Build history of the part. All positions in model axes, mm. A direction names the side the tool comes from. Round coordinates to 2 decimals unless told otherwise and drop trailing zeros. Write each loop counter-clockwise with the first axis right and the second up, starting at its lowest first coordinate (ties: lowest second). Pieces come first, ordered by that corner, then holes. Notation, with made-up numbers: M 11.25,80.5 L 21.25,80.5 A17 ccw 21.25,95.5 Z; hole C 19.25,-8.5 d8. An arc over 180 degrees is marked long. Write item = value, one per line. Start each with the question number.
Q1. Band-saw the part on A-A on x = -1.5. Write the cut outline in (y, z), plus the area to 3 significant figures.
Q2. Band-saw the part on C-C on x = 0. Write the cut outline in (y, z).
Q3. Band-saw the part on B-B on z = 3.5. Write the cut outline in (x, y), plus the area to 3 significant figures.
Q4. Tool access for faces 4 (the flat face through (4, 3.3, 5)), 5 (the flat face through (-4, 3.3, 5)), 6 (the cylindrical face through (2.747, 0.156, 4.934)): list every direction of +Z, -Z, +X, -X, +Y, -Y with a clear straight run to the whole face (end or side of a thin tool).
Q5. Probe L1, parallel to Z at x = 0, y = 1.75; L2, parallel to Z at x = 1.75, y = 1.3; L3, parallel to X at y = 3.85, z = 6.75. List the from-to ranges inside material, lowest first.
Q6. Pull direction Z, two halves, no side cores. Call faces 1 (the cylindrical face through (4.95, 2.37, 4.93)), 2 (the cylindrical face through (-1.5, 2.2, 1)), 3 (the cylindrical face through (3.894, 1.222, 0.086)): released by +Z, released by -Z, zero draft, split by the parting line, or undercut.
Q7. Band-saw the part on D-D on z = 9. Write the cut outline in (x, y), plus the area to 3 significant figures.
```python
from build123d import *

# Parameters (mm, degrees)
EXTRUDE_1_DEPTH     = 10
FILLET_3_R          = 0.3
SKETCH_2_R          = 2.5
CUT_EXTRUDE_1_DEPTH = 6


with BuildPart() as part:
    # 草图1 → 凸台-拉伸1 (new body)
    with BuildSketch(Plane.XY):
        with BuildLine():
            Line((-3, 4.3), (3, 4.3))
            Line((3, 4.3), (3, 3.8))
            ThreePointArc((3, 3.8), (3.146446609, 3.446446609), (3.5, 3.3))
            Line((3.5, 3.3), (5.1, 3.3))
            Line((5.1, 3.3), (5.1, 3.128427125))
            ThreePointArc((5.1, 3.128427125), (4.947759065, 2.36306026), (4.514213562, 1.714213562))
            Line((4.514213562, 1.714213562), (3.385786438, 0.585786438))
            ThreePointArc((3.385786438, 0.585786438), (2.73693974, 0.152240935), (1.971572875, 0))
            Line((1.971572875, 0), (-1.971572875, 0))
            ThreePointArc((-1.971572875, 0), (-2.73693974, 0.152240935), (-3.385786438, 0.585786438))
            Line((-3.385786438, 0.585786438), (-4.514213562, 1.714213562))
            ThreePointArc((-4.514213562, 1.714213562), (-4.947759065, 2.36306026), (-5.1, 3.128427125))
            Line((-5.1, 3.128427125), (-5.1, 3.3))
            Line((-5.1, 3.3), (-3.5, 3.3))
            ThreePointArc((-3.5, 3.3), (-3.146446609, 3.446446609), (-3, 3.8))
            Line((-3, 3.8), (-3, 4.3))
        make_face()
    extrude(amount=EXTRUDE_1_DEPTH)

    # 圆角3
    # the kernel refuses this fillet: 0.3 mm, written as the material it takes off along each edge
    with BuildSketch(Plane(origin=(-3, 3.8, 10), x_dir=(0, 0, -1), z_dir=(0, 1, 0)), Plane(origin=(3, 5.05, 10), x_dir=(0, 0, -1), z_dir=(0, -1, 0))) as fillet_3_piece_1:
        with BuildLine():
            CenterArc((FILLET_3_R, -FILLET_3_R), FILLET_3_R, 90, 90)
            Line((0, -FILLET_3_R), (0, 0))
            Line((0, 0), (FILLET_3_R, 0))
        make_face()
    extrude(amount=1.25, mode=Mode.SUBTRACT)
    with BuildSketch(Plane(origin=(3, 5.05, 0), x_dir=(0, 0, 1), z_dir=(0, -1, 0)), Plane(origin=(-3, 3.8, 0), x_dir=(0, 0, 1), z_dir=(0, 1, 0))) as fillet_3_piece_2:
        with BuildLine():
            CenterArc((FILLET_3_R, FILLET_3_R), FILLET_3_R, 180, 90)
            Line((0, FILLET_3_R), (0, 0))
            Line((0, 0), (FILLET_3_R, 0))
        make_face()
    extrude(amount=1.25, mode=Mode.SUBTRACT)
    with BuildSketch(Plane(origin=(4.514213562, 1.714213562, 10), x_dir=(0, 0, -1), z_dir=(-0.7071067811865436, -0.7071067811865515, 0)), Plane(origin=(-3.385786438, 0.585786438, 10), x_dir=(0, 0, -1), z_dir=(-0.7071067811865436, 0.7071067811865515, 0))) as fillet_3_piece_3:
        with BuildLine():
            CenterArc((FILLET_3_R, -FILLET_3_R), FILLET_3_R, 90, 90)
            Line((0, -FILLET_3_R), (0, 0))
            Line((0, 0), (FILLET_3_R, 0))
        make_face()
    extrude(amount=1.595836944, mode=Mode.SUBTRACT)
    with BuildSketch(Plane(origin=(1.971572875, 2, 10), x_dir=(0.7071067811865542, -0.7071067811865409, 0), z_dir=(0.7071067811865409, 0.7071067811865542, 0))) as fillet_3_piece_4:
        with BuildLine():
            CenterArc((2 - FILLET_3_R, FILLET_3_R), FILLET_3_R, 270, 90)
            Line((2 - FILLET_3_R, 0), (2, 0))
            Line((2, 0), (2, FILLET_3_R))
        make_face()
    revolve(axis=Axis((1.971572875, 2, 10), (0, 0, -1)), revolution_arc=45, mode=Mode.SUBTRACT)
    with BuildSketch(Plane(origin=(1.971572875, 0, 10), x_dir=(0, 0, -1), z_dir=(-1, 0, 0))) as fillet_3_piece_5:
        with BuildLine():
            CenterArc((FILLET_3_R, -FILLET_3_R), FILLET_3_R, 90, 90)
            Line((0, -FILLET_3_R), (0, 0))
            Line((0, 0), (FILLET_3_R, 0))
        make_face()
    extrude(amount=3.943145751, mode=Mode.SUBTRACT)
    with BuildSketch(Plane(origin=(-1.971572875, 2, 10), x_dir=(0, -1, 0), z_dir=(1, 0, 0))) as fillet_3_piece_6:
        with BuildLine():
            CenterArc((2 - FILLET_3_R, FILLET_3_R), FILLET_3_R, 270, 90)
            Line((2 - FILLET_3_R, 0), (2, 0))
            Line((2, 0), (2, FILLET_3_R))
        make_face()
    revolve(axis=Axis((-1.971572875, 2, 10), (0, 0, -1)), revolution_arc=45, mode=Mode.SUBTRACT)
    with BuildSketch(Plane(origin=(-3.1, 3.128427125, 10), x_dir=(-0.7071067811865485, -0.7071067811865466, 0), z_dir=(0.7071067811865466, -0.7071067811865485, 0))) as fillet_3_piece_7:
        with BuildLine():
            CenterArc((2 - FILLET_3_R, FILLET_3_R), FILLET_3_R, 270, 90)
            Line((2 - FILLET_3_R, 0), (2, 0))
            Line((2, 0), (2, FILLET_3_R))
        make_face()
    revolve(axis=Axis((-3.1, 3.128427125, 10), (0, 0, -1)), revolution_arc=45, mode=Mode.SUBTRACT)
    with BuildSketch(Plane(origin=(-5.85, 3.3, 10), x_dir=(0, 0, -1), z_dir=(1, 0, 0)), Plane(origin=(3.5, 3.3, 10), x_dir=(0, 0, -1), z_dir=(1, 0, 0))) as fillet_3_piece_8:
        with BuildLine():
            CenterArc((FILLET_3_R, -FILLET_3_R), FILLET_3_R, 90, 90)
            Line((0, -FILLET_3_R), (0, 0))
            Line((0, 0), (FILLET_3_R, 0))
        make_face()
    extrude(amount=2.35, mode=Mode.SUBTRACT)
    with BuildSketch(Plane(origin=(-3.5, 3.8, 10), x_dir=(0, -1, 0), z_dir=(-1, 0, 0))) as fillet_3_piece_9:
        with BuildLine():
            CenterArc((0.5 + FILLET_3_R, -FILLET_3_R), FILLET_3_R, 90, 90)
            Line((0.5 + FILLET_3_R, 0), (0.5, 0))
            Line((0.5, 0), (0.5, -FILLET_3_R))
        make_face()
    revolve(axis=Axis((-3.5, 3.8, 10), (0, 0, 1)), revolution_arc=90, mode=Mode.SUBTRACT)
    with BuildSketch(Plane(origin=(3.5, 3.3, 0), x_dir=(0, 0, 1), z_dir=(1, 0, 0)), Plane(origin=(-5.85, 3.3, 0), x_dir=(0, 0, 1), z_dir=(1, 0, 0))) as fillet_3_piece_10:
        with BuildLine():
            CenterArc((FILLET_3_R, FILLET_3_R), FILLET_3_R, 180, 90)
            Line((0, FILLET_3_R), (0, 0))
            Line((0, 0), (FILLET_3_R, 0))
        make_face()
    extrude(amount=2.35, mode=Mode.SUBTRACT)
    with BuildSketch(Plane(origin=(3.5, 3.8, 0), x_dir=(-1, 0, 0), z_dir=(0, 1, 0))) as fillet_3_piece_11:
        with BuildLine():
            CenterArc((0.5 + FILLET_3_R, FILLET_3_R), FILLET_3_R, 180, 90)
            Line((0.5 + FILLET_3_R, 0), (0.5, 0))
            Line((0.5, 0), (0.5, FILLET_3_R))
        make_face()
    revolve(axis=Axis((3.5, 3.8, 0), (0, 0, 1)), revolution_arc=90, mode=Mode.SUBTRACT)
    with BuildSketch(Plane(origin=(-3.385786438, 0.585786438, 0), x_dir=(0, 0, 1), z_dir=(-0.7071067811865436, 0.7071067811865515, 0)), Plane(origin=(4.514213562, 1.714213562, 0), x_dir=(0, 0, 1), z_dir=(-0.7071067811865436, -0.7071067811865515, 0))) as fillet_3_piece_12:
        with BuildLine():
            CenterArc((FILLET_3_R, FILLET_3_R), FILLET_3_R, 180, 90)
            Line((0, FILLET_3_R), (0, 0))
            Line((0, 0), (FILLET_3_R, 0))
        make_face()
    extrude(amount=1.595836944, mode=Mode.SUBTRACT)
    with BuildSketch(Plane(origin=(-1.971572875, 2, 0), x_dir=(0, -1, 0), z_dir=(1, 0, 0))) as fillet_3_piece_13:
        with BuildLine():
            CenterArc((2 - FILLET_3_R, -FILLET_3_R), FILLET_3_R, 0, 90)
            Line((2 - FILLET_3_R, 0), (2, 0))
            Line((2, 0), (2, -FILLET_3_R))
        make_face()
    revolve(axis=Axis((-1.971572875, 2, 0), (0, 0, -1)), revolution_arc=45, mode=Mode.SUBTRACT)
    with BuildSketch(Plane(origin=(1.971572875, 0, 0), x_dir=(0, 0, 1), z_dir=(-1, 0, 0))) as fillet_3_piece_14:
        with BuildLine():
            CenterArc((FILLET_3_R, FILLET_3_R), FILLET_3_R, 180, 90)
            Line((0, FILLET_3_R), (0, 0))
            Line((0, 0), (FILLET_3_R, 0))
        make_face()
    extrude(amount=3.943145751, mode=Mode.SUBTRACT)
    with BuildSketch(Plane(origin=(1.971572875, 2, 0), x_dir=(0.7071067811865542, -0.7071067811865409, 0), z_dir=(0.7071067811865409, 0.7071067811865542, 0))) as fillet_3_piece_15:
        with BuildLine():
            CenterArc((2 - FILLET_3_R, -FILLET_3_R), FILLET_3_R, 0, 90)
            Line((2 - FILLET_3_R, 0), (2, 0))
            Line((2, 0), (2, -FILLET_3_R))
        make_face()
    revolve(axis=Axis((1.971572875, 2, 0), (0, 0, -1)), revolution_arc=45, mode=Mode.SUBTRACT)
    with BuildSketch(Plane(origin=(3.1, 3.128427125, 0), x_dir=(1, 0, 0), z_dir=(0, 1, 0))) as fillet_3_piece_16:
        with BuildLine():
            CenterArc((2 - FILLET_3_R, -FILLET_3_R), FILLET_3_R, 0, 90)
            Line((2 - FILLET_3_R, 0), (2, 0))
            Line((2, 0), (2, -FILLET_3_R))
        make_face()
    revolve(axis=Axis((3.1, 3.128427125, 0), (0, 0, -1)), revolution_arc=45, mode=Mode.SUBTRACT)
    with BuildSketch(Plane(origin=(3.1, 3.128427125, 10), x_dir=(1, 0, 0), z_dir=(0, 1, 0))) as fillet_3_piece_17:
        with BuildLine():
            CenterArc((2 - FILLET_3_R, FILLET_3_R), FILLET_3_R, 270, 90)
            Line((2 - FILLET_3_R, 0), (2, 0))
            Line((2, 0), (2, FILLET_3_R))
        make_face()
    revolve(axis=Axis((3.1, 3.128427125, 10), (0, 0, -1)), revolution_arc=45, mode=Mode.SUBTRACT)
    with BuildSketch(Plane(origin=(-3.1, 3.128427125, 0), x_dir=(-0.7071067811865485, -0.7071067811865466, 0), z_dir=(0.7071067811865466, -0.7071067811865485, 0))) as fillet_3_piece_18:
        with BuildLine():
            CenterArc((2 - FILLET_3_R, -FILLET_3_R), FILLET_3_R, 0, 90)
            Line((2 - FILLET_3_R, 0), (2, 0))
            Line((2, 0), (2, -FILLET_3_R))
        make_face()
    revolve(axis=Axis((-3.1, 3.128427125, 0), (0, 0, -1)), revolution_arc=45, mode=Mode.SUBTRACT)
    with BuildSketch(Plane(origin=(3.5, 3.8, 10), x_dir=(-1, 0, 0), z_dir=(0, 1, 0))) as fillet_3_piece_19:
        with BuildLine():
            CenterArc((0.5 + FILLET_3_R, -FILLET_3_R), FILLET_3_R, 90, 90)
            Line((0.5 + FILLET_3_R, 0), (0.5, 0))
            Line((0.5, 0), (0.5, -FILLET_3_R))
        make_face()
    revolve(axis=Axis((3.5, 3.8, 10), (0, 0, 1)), revolution_arc=90, mode=Mode.SUBTRACT)
    with BuildSketch(Plane(origin=(-3.5, 3.8, 0), x_dir=(0, -1, 0), z_dir=(-1, 0, 0))) as fillet_3_piece_20:
        with BuildLine():
            CenterArc((0.5 + FILLET_3_R, FILLET_3_R), FILLET_3_R, 180, 90)
            Line((0.5 + FILLET_3_R, 0), (0.5, 0))
            Line((0.5, 0), (0.5, FILLET_3_R))
        make_face()
    revolve(axis=Axis((-3.5, 3.8, 0), (0, 0, 1)), revolution_arc=90, mode=Mode.SUBTRACT)
    with BuildSketch(Plane(origin=(-5.1, 3.128427125, 0), x_dir=(0, 0, 1), z_dir=(0, 1, 0)), Plane(origin=(5.1, 4.05, 0), x_dir=(0, 0, 1), z_dir=(0, -1, 0))) as fillet_3_piece_21:
        with BuildLine():
            CenterArc((FILLET_3_R, FILLET_3_R), FILLET_3_R, 180, 90)
            Line((0, FILLET_3_R), (0, 0))
            Line((0, 0), (FILLET_3_R, 0))
        make_face()
    extrude(amount=0.921572875, mode=Mode.SUBTRACT)
    with BuildSketch(Plane(origin=(5.1, 4.05, 10), x_dir=(0, 0, -1), z_dir=(0, -1, 0)), Plane(origin=(-5.1, 3.128427125, 10), x_dir=(0, 0, -1), z_dir=(0, 1, 0))) as fillet_3_piece_22:
        with BuildLine():
            CenterArc((FILLET_3_R, -FILLET_3_R), FILLET_3_R, 90, 90)
            Line((0, -FILLET_3_R), (0, 0))
            Line((0, 0), (FILLET_3_R, 0))
        make_face()
    extrude(amount=0.921572875, mode=Mode.SUBTRACT)

    # 草图2 → 切除-拉伸1 (cut)
    with BuildSketch(Plane(origin=(0, 4.3, 0), x_dir=(1, 0, 0), z_dir=(0, 1, 0))):
        with Locations(Location((0, -3, 0), (0, 0, 270))):
            Circle(SKETCH_2_R)
    extrude(amount=-CUT_EXTRUDE_1_DEPTH, mode=Mode.SUBTRACT)


solid = part.part
```
Conclusion:
q1.outline = M 0,0.3 A0.3 ccw 0.3,0 L 4.3,0 L 4.3,1 L 0,1 Z; M 0,5 L 4.3,5 L 4.3,10 L 0.3,10 A0.3 ccw 0,9.7 Z
q1.area = 25.8 mm^2
q2.outline = M 0,0.3 A0.3 ccw 0.3,0 L 4.3,0 L 4.3,0.5 L 0,0.5 Z; M 0,5.5 L 4.3,5.5 L 4.3,10 L 0.3,10 A0.3 ccw 0,9.7 Z
q3.outline = M -5.1,3.13 A2 ccw -4.51,1.71 L -3.39,0.59 A2 ccw -2.45,0.06 L -2.45,4.3 L -3,4.3 L -3,3.8 A0.5 cw -3.5,3.3 L -5.1,3.3 Z; M 2.45,0.06 A2 ccw 3.39,0.59 L 4.51,1.71 A2 ccw 5.1,3.13 L 5.1,3.3 L 3.5,3.3 A0.5 cw 3,3.8 L 3,4.3 L 2.45,4.3 Z
q3.area = 13.1 mm^2
q4.face_4 = +Z, -Z, +X, +Y
q4.face_5 = +Z, -Z, -X, +Y
q4.face_6 = +Z, -Z, +X, -Y
q5.L1 = 0 to 0.5, 5.5 to 10
q5.L2 = 0 to 1.21, 4.79 to 10
q5.L3 = -3 to 3
q6.face_1 = zero draft
q6.face_2 = undercut
q6.face_3 = released by -Z
q7.outline = M -5.1,3.13 A2 ccw -4.51,1.71 L -3.39,0.59 A2 ccw -1.97,0 L 1.97,0 A2 ccw 3.39,0.59 L 4.51,1.71 A2 ccw 5.1,3.13 L 5.1,3.3 L 3.5,3.3 A0.5 cw 3,3.8 L 3,4.3 L -3,4.3 L -3,3.8 A0.5 cw -3.5,3.3 L -5.1,3.3 Z
q7.area = 34.1 mm^2
